CAD build for the part. Positions are in the model's coordinates, mm. A direction names the side the tool comes from. Give positions to 0.01 mm unless a question says otherwise; leave off trailing zeros. Write each loop counter-clockwise with the first axis right and the second up, starting at its lowest first coordinate (ties: lowest second). Pieces come first, ordered by that corner, then holes. Notation, with made-up numbers: (20, 18.25) - (63, 18.25) arc R17 ccw to (63, 51.25) - close; hole circle Ø8 at (58, 57.5). An arc over 180 degrees is marked (long way). Answer as a JSON object with one key per item and string values.
from build123d import *

# Parameters (mm, degrees)
CROQUIS1_W              = 5
CROQUIS1_H              = 30
SALIENTE_EXTRUIR1_DEPTH = 4
SALIENTE_EXTRUIR2_START = 4
CROQUIS2_R              = 10
CROQUIS2_R_2            = 4.15
SALIENTE_EXTRUIR2_DEPTH = 25
CORTAR_EXTRUIR1_START   = 4
CROQUIS3_R              = 4.15
CORTAR_EXTRUIR1_DEPTH   = 4
CROQUIS4_R              = 2
CORTAR_EXTRUIR2_DEPTH   = 29


with BuildPart() as part:
    # Croquis1 → Saliente-Extruir1 (new body)
    with BuildSketch(Plane.XY):
        with BuildLine():
            Line((10, -18), (10, 28))
            Line((10, 28), (-10, 28))
            Line((-10, 28), (-10, -18))
            ThreePointArc((-10, -18), (0, -28), (10, -18))
        make_face()
        with Locations((0, 10)):
            Rectangle(CROQUIS1_W, CROQUIS1_H, mode=Mode.SUBTRACT)
    extrude(amount=SALIENTE_EXTRUIR1_DEPTH)

    # Croquis2 → Saliente-Extruir2 (add)
    with BuildSketch(Plane.XY.offset(SALIENTE_EXTRUIR2_START)):
        with Locations((0, -18)):
            Circle(CROQUIS2_R)
        with Locations((0, -18)):
            Circle(CROQUIS2_R_2, mode=Mode.SUBTRACT)
    extrude(amount=SALIENTE_EXTRUIR2_DEPTH)

    # Croquis3 → Cortar-Extruir1 (cut)
    with BuildSketch(Plane.XY.offset(CORTAR_EXTRUIR1_START)):
        with Locations((0, -18)):
            Circle(CROQUIS3_R)
    extrude(amount=-CORTAR_EXTRUIR1_DEPTH, mode=Mode.SUBTRACT)

    # Croquis4 → Cortar-Extruir2 (cut, through all)
    with BuildSketch(Plane(origin=(0, 0, 0), x_dir=(1, 0, 0), z_dir=(0, 1, 0))):
        with Locations((0, -10)):
            Circle(CROQUIS4_R)
        with Locations((0, -22.5)):
            Circle(CROQUIS4_R)
    extrude(amount=-CORTAR_EXTRUIR2_DEPTH, mode=Mode.SUBTRACT)


solid = part.part
Item 1: Cut at C-C (z = 22.5). Give the cut face in (x, y), and give its area (3 significant figures).
Entries:
{"outline": "(-2, -27.8) - (-2, -21.64) arc R4.15 cw to (-2, -14.36) - (-2, -8.2) arc R10 ccw to start; (2, -27.8) arc R10 ccw to (2, -8.2) - (2, -14.36) arc R4.15 cw to (2, -21.64) - close", "area": "212 mm2"}
Item 2: Cut at A-A (y = 24). Give the cut face in (x, z).
Entries:
{"outline": "(-10, 0) - (-2.5, 0) - (-2.5, 4) - (-10, 4) - close; (2.5, 0) - (10, 0) - (10, 4) - (2.5, 4) - close"}
Item 3: Cut at B-B (x = 0). State how many separate pieces and enclosed holes the cut face has, and give its area (3 significant figures).
Entries:
{"separate pieces": "7", "enclosed holes": "0", "area": "270 mm2"}
Item 4: Which spindle directions (+Z, -Z, +X, -X, +Y, -Y) get a long thin tool onto all of the face, cutting with end or side? Do faces 1 (the flat face through (2.5, 10, 2)), 2 (the flat face through (0, 28, 2)), 3 (the cylindrical face through (-2.17, -27.76, 14.3)). Say none if no direction does.
Entries:
{"face 1": "+Z, -Z", "face 2": "+Z, -Z, +X, -X, +Y", "face 3": "+Z"}
Item 5: Probe line 1 (Z direction, x = 0, y = -9.75); line 2 (X direction, y = -24, z = 22.5); line 3 (Y direction, x = 3.25, z = 3.25). List the from-to ranges inside material, lowest first. Write a range as from..to.
Entries:
{"line 1": "0..8, 12..20.5, 24.5..29", "line 2": "-8..-2, 2..8", "line 3": "-27.46..-20.58, -15.42..28"}
Item 6: Flat gauge pins, fed straight in: P1, Ø2, axis at x = -0.5, y = 17, coming from the -Z side; P2, Ø2, axis at x = 6, z = 11.5, coming from the -Y side; P3, Ø6, axis at x = -3.5, y = 11, coming from the +Z side; P4, Ø1.5, axis at x = -5.5, z = 12.5, coming from the -Y side. Where does each tip first touch, or does it go through?
Entries:
{"P1": "through", "P2": "y = -26.66", "P3": "z = 4", "P4": "y = -26.8"}
Item 7: Cut at D-D (x = 3.5). Give the cut face in (y, z), and give its area (3 significant figures).
Entries:
{"outline": "(-27.37, 0) - (-20.23, 0) - (-20.23, 29) - (-27.37, 29) - close; (-15.77, 0) - (28, 0) - (28, 4) - (-8.63, 4) - (-8.63, 29) - (-15.77, 29) - close", "area": "561 mm2"}
Item 8: Mould opens along X. For faces 4 (the cylindrical face through (-1.998, -24.776, 22.412)), 5 (the flat face through (-10, 5, 2)), 6 (the flat face through (-0.1, -22.3, 29)) say: +X half, -X half, draft (parallel to the pull), parting line (faces both ways), or undercut.
Entries:
{"face 4": "undercut", "face 5": "-X half", "face 6": "draft"}
